Check sheet for the modelled part. Datum: model origin and axes. Units: mm. Face numbers are marked on the shaded views. A direction names the side the tool comes from. Round coordinates to 2 decimals unless told otherwise and drop trailing zeros. Loops run counter-clockwise (first coordinate to the right, second up) from the corner with the lowest first, then second, coordinate; pieces in that order, holes last. Notation, with made-up numbers: M 12.5,36.25 L 35.5,36.25 A19 cw 35.5,47.25 Z; hole C -21,-18 d4. An arc over 180 degrees is marked long. Write item = value, one per line. Start each with the question number.
(1) Go/stop test with flat-tipped pins: P1, Ø2, axis at y = -2, z = 0, coming from the +X side; P2, Ø1.8, axis at y = -1, z = 0, coming from the -X side; P3, Ø3.5, axis at x = 0.5, y = 0.5, coming from the +Z side. Record where each tip stops, or that it passes through.
(2) Scan lines: L1, parallel to X at y = -3.5, z = 1.75; L2, parallel to Y at x = 0.5, z = 6.75; L3, parallel to Z at x = -3.25, y = 3.75. Record each from-to range of solid material in increasing order. Write a range as from..to.
(3) Cross-section at D-D on y = 6.25. Record the boundary of the cut face in (x, z).
(4) Set-up check for the marked faces 5, 6 and 7: record each of +Z, -Z, +X, -X, +Y, -Y from which the full face is reachable in a straight line by a thin tool's end or side.
(5) Cross-section at B-B on y = 0.75. Record the boundary of the cut face in (x, z).
(6) Cross-section at C-C on y = -6. Record the boundary of the cut face in (x, z), plus the area to 3 significant figures.
(7) Mould release check, pull along Y, two halves, no side actions. Record for the marked faces 1, 2, 3 and 4: pulls with the +Y half, pulls with the -Y half, needs draft (parallel to the pull), parting line crosses it, or undercut.
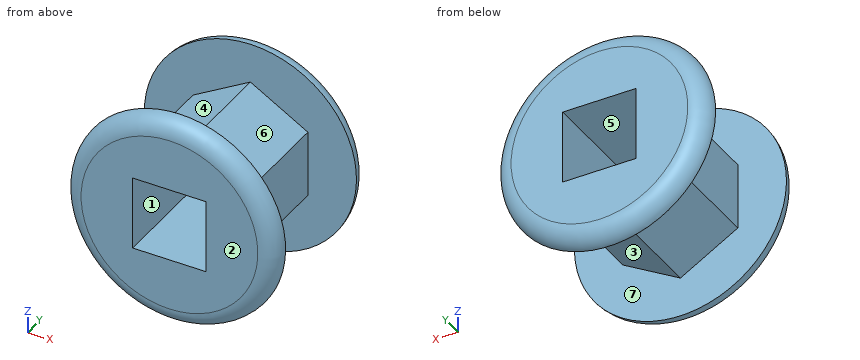
from build123d import *

# Parameters (mm, degrees)
BOSS_EXTRUDE1_DEPTH = 6.35
SKETCH2_R           = 9.525
BOSS_EXTRUDE2_DEPTH = 0.79375
SKETCH3_W           = 6.604
SKETCH3_H           = 6.604
CUT_EXTRUDE1_DEPTH  = 20.636290542
FILLET1_R           = 1.5875


with BuildPart() as part:
    # Sketch1 → Boss-Extrude1 (new, symmetric)
    with BuildSketch(Plane(origin=(0, 0, 0), x_dir=(1, 0, 0), z_dir=(0, 1, 0))):
        Polygon((0, 5.95753309), (-5.159375, 2.978766545), (-5.159375, -2.978766545), (0, -5.95753309), (5.159375, -2.978766545), (5.159375, 2.978766545), align=None)
    extrude(amount=BOSS_EXTRUDE1_DEPTH, both=True)

    # Sketch2 → Boss-Extrude2 (add, symmetric)
    with BuildSketch(Plane(origin=(0, 6.35, 0), x_dir=(1, 0, 0), z_dir=(0, 1, 0))):
        with Locations(Location((0, 0, 0), (0, 0, 270))):
            Circle(SKETCH2_R)
    boss_extrude2 = extrude(amount=BOSS_EXTRUDE2_DEPTH, both=True)

    # Mirror1: Boss-Extrude2 across plane
    add(boss_extrude2.mirror(Plane.ZX))

    # Sketch3 → Cut-Extrude1 (cut, through all)
    with BuildSketch(Plane(origin=(0, 7.14375, 0), x_dir=(1, 0, 0), z_dir=(0, 1, 0))):
        Rectangle(SKETCH3_W, SKETCH3_H)
    extrude(amount=-CUT_EXTRUDE1_DEPTH, mode=Mode.SUBTRACT)

    # Fillet1
    fillet1_edges = [part.edges().sort_by_distance(p)[0] for p in [
        (0, 7.14375, -9.525),
        (0, -7.14375, -9.525),
    ]]
    fillet(fillet1_edges, radius=FILLET1_R - 0.0001)  # a hair under: the kernel refuses the full size


solid = part.part
Result:
q1.P1 = 5.16
q1.P2 = -5.16
q1.P3 = 5.96
q2.L1 = -5.16..-3.3, 3.3..5.16
q2.L2 = -7.14..-5.56, 5.56..7.14
q2.L3 = -4.08..-3.3, 3.3..4.08
q3.outline = C 0,0 d18.73; hole M -3.3,-3.3 L 3.3,-3.3 L 3.3,3.3 L -3.3,3.3 Z
q4.face_5 = +Y, -Y
q4.face_6 = +Z, +X
q4.face_7 = none
q5.outline = M -5.16,-2.98 L 0,-5.96 L 5.16,-2.98 L 5.16,2.98 L 0,5.96 L -5.16,2.98 Z; hole M -3.3,-3.3 L 3.3,-3.3 L 3.3,3.3 L -3.3,3.3 Z
q6.outline = C 0,0 d18.92; hole M -3.3,-3.3 L 3.3,-3.3 L 3.3,3.3 L -3.3,3.3 Z
q6.area = 238 mm^2
q7.face_1 = needs draft
q7.face_2 = pulls with the -Y half
q7.face_3 = undercut
q7.face_4 = undercut
